Can you work these out from the drawing? Everything is in mm from the part's minimum corner. Give positions to 0.01 mm unless a question says otherwise; leave off trailing zeros. Write each loop counter-clockwise with the first axis right and the second up, starting at its lowest first coordinate (ties: lowest second). Pieces come first, ordered by that corner, then holes. Notation, with made-up numbers: (-22, 66.25) -> (-5, 66.25) arc R31 ccw to (-5, 105.25) -> close; hole circle Ø3 at (-27.75, 2). An arc over 180 degrees is marked (long way). Return JSON: item names as keys, results as strings.
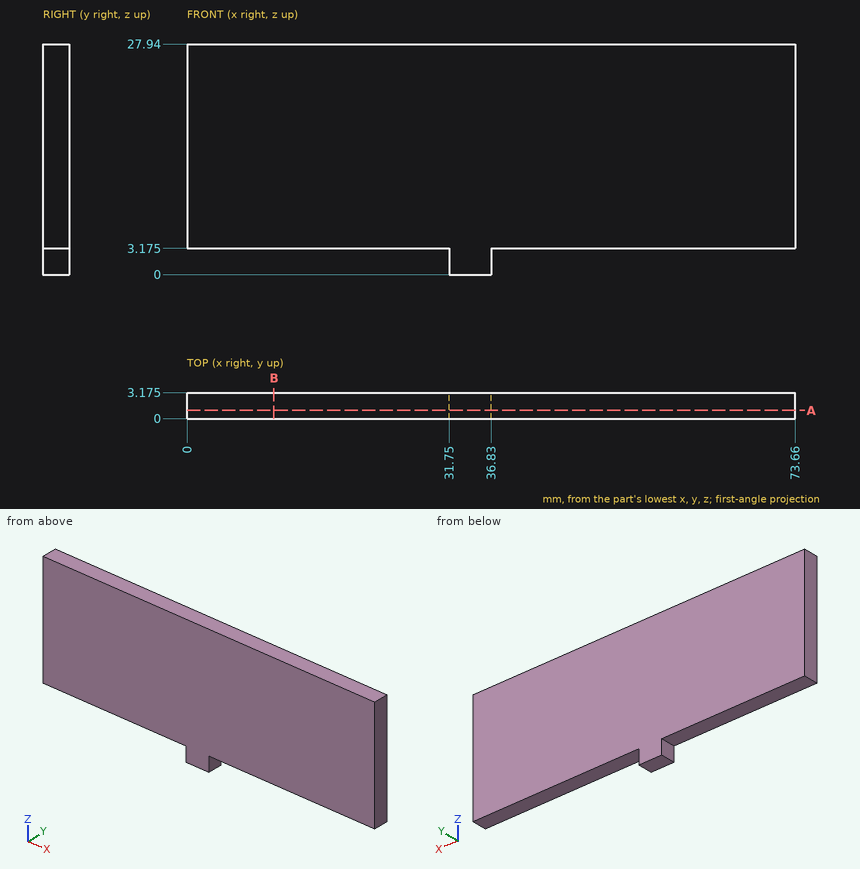
1. Suppose I cut it at B-B, the plane x = 10.5. List the corners of the cut face in (y, z) for me (3 decimals).
Taken from the geometry:
{"outline": "(0, 3.175) -> (3.175, 3.175) -> (3.175, 27.94) -> (0, 27.94) -> close"}
2. Suppose I cut it at A-A, the plane y = 1. List the corners of the cut face in (x, z) for me (3 decimals), and give its area (3 significant figures).
Taken from the geometry:
{"outline": "(0, 3.175) -> (31.75, 3.175) -> (31.75, 0) -> (36.83, 0) -> (36.83, 3.175) -> (73.66, 3.175) -> (73.66, 27.94) -> (0, 27.94) -> close", "area": "1,840 mm²"}
3. If I drill on line 1 (Z direction, x = 25, y = 1) (3 decimals); line 2 (X direction, y = 2.85, z = 3), over which ranges is the centre line in solid material (lowest first)? Write a range as [from, to].
Taken from the geometry:
{"line 1": "z = [3.175, 27.94]", "line 2": "x = [31.75, 36.83]"}
4. For pin 1 Ø1.6 at (y, z) = (1, 1) entering from -X; pin 2 Ø2 at (x, z) = (39, 13) entering from -Y; pin 3 Ø1 at (y, z) = (1.5, 2.5) entering from +X, each with a flat end and sliding along its axis, tell me the tip position at first contact or that it passes through.
Taken from the geometry:
{"pin 1": "stops at x = 31.75", "pin 2": "stops at y = 0", "pin 3": "stops at x = 36.83"}
